Geometry: final body of the model. Coordinates: model frame, mm. A direction names the side the tool comes from. Round coordinates to 2 decimals unless told otherwise and drop trailing zeros. Write each loop counter-clockwise with the first axis right and the second up, starting at its lowest first coordinate (ties: lowest second). Pieces come first, ordered by that corner, then holes. Notation, with made-up numbers: M 32,-18 L 69,-18 A17 cw 69,-8 Z; hole C 59.25,43.5 d9. An arc over 180 degrees is marked long. Use one line per item in the form item = value. Start each with the question number.
Item 1: Pull-direction query (Z, two-part tool) for faces 1 (the flat face through (0, -11, 5)), 2 (the flat face through (10, 0, 13)), 3 (the flat face through (-5, 0, 0)); classes: pulls with the +Z half, pulls with the -Z half, needs draft (parallel to the pull), parting line crosses it, or undercut.
Item 2: Section query A-A (y = 0). Return loops of the section in (x, z), and give its area (3 significant figures).
Item 3: Reachability of faces 4 (the flat face through (8, 0, 12)), 5 (the flat face through (10, 0, 11)), 6 (the flat face through (0, 8, 12)), 7 (the flat face through (0, -8, 12)), 8 (the flat face through (-8, 0, 12)) from +Z, -Z, +X, -X, +Y, -Y: full face, straight path, thin tool, end or side. Return the list, or none.
Item 4: Pin query (flat end, axial travel): pin 1 Ø1 at (x, z) = (0, 12) entering from +Y; pin 2 Ø10 at (y, z) = (-1.5, -19.5) entering from -X; pin 3 Ø4 at (x, y) = (-1, -7) entering from -Z. Return the tip coordinate at first contact, or that it passes through.
Item 5: Ray query, probe 1 along Z at (x, y) = (5.75, -8.25); probe 2 along Z at (x, y) = (-6.25, 3.5); probe 3 along Y at (x, z) = (-0.25, -41). Return the intervals inside material, ascending.
Item 6: Section query C-C (z = -47). Return loops of the section in (x, y), and give its area (3 significant figures).
from build123d import *

# Parameters (mm, degrees)
SKETCH1_W           = 22
SKETCH1_H           = 22
BOSS_EXTRUDE1_DEPTH = 24
SKETCH2_W           = 2
SKETCH2_H           = 22
CUT_EXTRUDE1_DEPTH  = 3
CIRPATTERN1_COUNT   = 4
FILLET1_R           = 1
SKETCH3_R           = 4
BOSS_EXTRUDE2_DEPTH = 60


with BuildPart() as part:
    # Sketch1 → Boss-Extrude1 (new body)
    with BuildSketch(Plane.XY):
        Rectangle(SKETCH1_W, SKETCH1_H)
    extrude(amount=BOSS_EXTRUDE1_DEPTH)

    # Sketch2 → Cut-Extrude1 (cut)
    with BuildSketch(Plane(origin=(11, 0, 0), x_dir=(0, 0, -1), z_dir=(1, 0, 0))):
        with Locations((-12, 0)):
            Rectangle(SKETCH2_W, SKETCH2_H)
    cut_extrude1 = extrude(amount=-CUT_EXTRUDE1_DEPTH, mode=Mode.SUBTRACT)

    # CirPattern1: Cut-Extrude1 ×4 about axis
    cirpattern1_axis = Axis((0, 0, 0), (0, 0, 1))
    for i in range(1, CIRPATTERN1_COUNT):
        add(cut_extrude1.rotate(cirpattern1_axis, i * 360 / CIRPATTERN1_COUNT), mode=Mode.SUBTRACT)

    # Fillet1
    fillet1_edges = [part.edges().sort_by_distance(p)[0] for p in [
        (11, -11, 5.5),
        (11, 11, 5.5),
        (-11, -11, 5.5),
        (-11, 11, 5.5),
        (11, -11, 18.5),
        (-11, -11, 18.5),
        (-11, 11, 18.5),
        (11, 11, 18.5),
    ]]
    fillet(fillet1_edges, radius=FILLET1_R)

    # Sketch3 → Boss-Extrude2 (add)
    with BuildSketch(Plane.XY):
        Circle(SKETCH3_R)
    extrude(amount=-BOSS_EXTRUDE2_DEPTH)


solid = part.part
Working result:
q1.face_1 = needs draft
q1.face_2 = undercut
q1.face_3 = pulls with the -Z half
q2.outline = M -11,0 L -4,0 L -4,-60 L 4,-60 L 4,0 L 11,0 L 11,11 L 8,11 L 8,13 L 11,13 L 11,24 L -11,24 L -11,13 L -8,13 L -8,11 L -11,11 Z
q2.area = 996 mm²
q3.face_4 = +X, +Y, -Y
q3.face_5 = none
q3.face_6 = +X, -X, +Y
q3.face_7 = +X, -X, -Y
q3.face_8 = -X, +Y, -Y
q4.pin_1 = 8
q4.pin_2 = -4
q4.pin_3 = 0
q5.probe_1 = 0 to 11, 13 to 24
q5.probe_2 = 0 to 24
q5.probe_3 = -3.99 to 3.99
q6.outline = C 0,0 d8
q6.area = 50.3 mm²
